Can you work these out from the drawing? Everything is in mm from the part's minimum corner. A direction names the side the tool comes from. Coordinates: 2 decimals unless noted, no trailing zeros. Loops run counter-clockwise (first coordinate to the right, second up) from the corner with the lowest first, then second, coordinate; pieces in that order, holes last. Notation, with made-up numbers: (69.5, 56) -> (75.5, 56) arc R33 cw to (75.5, 94) -> close; hole circle Ø4 at (56.25, 87). An arc over 180 degrees is marked (long way). One line per question, with ' | ' between items.
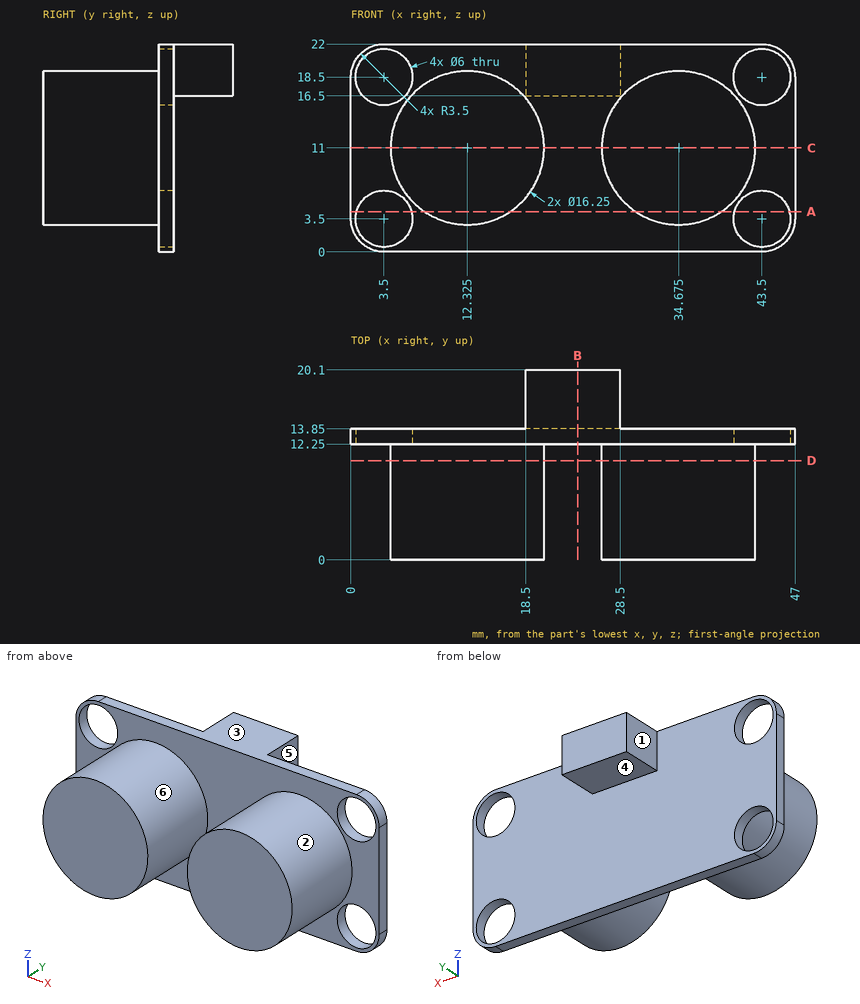
Q1. We'd pull the mould along X, two halves only. Please class the marked faces 4, 5 and 6: released by +X, released by -X, zero draft, split by the parting line, or undercut.
Values follow:
face 4: zero draft | face 5: released by +X | face 6: undercut
Q2. Imagine slicing it at A-A on z = 4.25. Write out the boundary of the cut face in (x, y).
Values follow:
outline: (0, 12.25) -> (0.6, 12.25) -> (0.6, 13.85) -> (0, 13.85) -> close; (6.4, 12.25) -> (7.8, 12.25) -> (7.8, 0) -> (16.85, 0) -> (16.85, 12.25) -> (30.15, 12.25) -> (30.15, 0) -> (39.2, 0) -> (39.2, 12.25) -> (40.6, 12.25) -> (40.6, 13.85) -> (6.4, 13.85) -> close; (46.4, 12.25) -> (47, 12.25) -> (47, 13.85) -> (46.4, 13.85) -> close
Q3. Imagine slicing it at B-B on x = 24. Write out the boundary of the cut face in (y, z), plus the area to 3 significant figures.
Values follow:
outline: (12.25, 0) -> (13.85, 0) -> (13.85, 16.5) -> (20.1, 16.5) -> (20.1, 22) -> (12.25, 22) -> close | area: 69.6 mm2
Q4. Please list where these lines run through material, in increasing order: L1, parallel to X at y = 13.1, z = 18.5; L2, parallel to Y at x = 32.5, z = 8.75; L3, parallel to Y at x = 44, z = 10. Write a range as [from, to].
Values follow:
L1: x = [0, 0.5], [6.5, 40.5], [46.5, 47] | L2: y = [0, 13.85] | L3: y = [12.25, 13.85]
Q5. For pin 1 (8 mm diameter, centred on x = 22, z = 5.5, fed in from +Y); pin 2 (1 mm diameter, centred on y = 8.5, z = 19, fed in from -X); pin 3 (3 mm diameter, centred on x = 26, z = 19, fed in from -Y); pin 4 (3.5 mm diameter, centred on x = 43.5, z = 18.5, fed in from +Y), each with a flat end and sliding along its axis, tell me the tip position at first contact or that it passes through.
Values follow:
pin 1: stops at y = 13.85 | pin 2: stops at x = 9.2 | pin 3: stops at y = 12.25 | pin 4: passes through
Q6. For the marked faces 1, 2 and 3, which set-ups out of +Z, -Z, +X, -X, +Y, -Y let a thin tool reach every point of the face, with its end or its side?
Values follow:
face 1: +Z, -Z, -X, +Y | face 2: -Y | face 3: +Z, +X, -X, +Y, -Y
Q7. Imagine slicing it at C-C on z = 11. Write out the boundary of the cut face in (x, y), plus the area to 3 significant figures.
Values follow:
outline: (0, 12.25) -> (4.2, 12.25) -> (4.2, 0) -> (20.45, 0) -> (20.45, 12.25) -> (26.55, 12.25) -> (26.55, 0) -> (42.8, 0) -> (42.8, 12.25) -> (47, 12.25) -> (47, 13.85) -> (0, 13.85) -> close | area: 473 mm2
Q8. Imagine slicing it at D-D on y = 10.5. Write out the boundary of the cut face in (x, z) (3 decimals).
Values follow:
outline: circle Ø16.25 at (12.325, 11); circle Ø16.25 at (34.675, 11)
